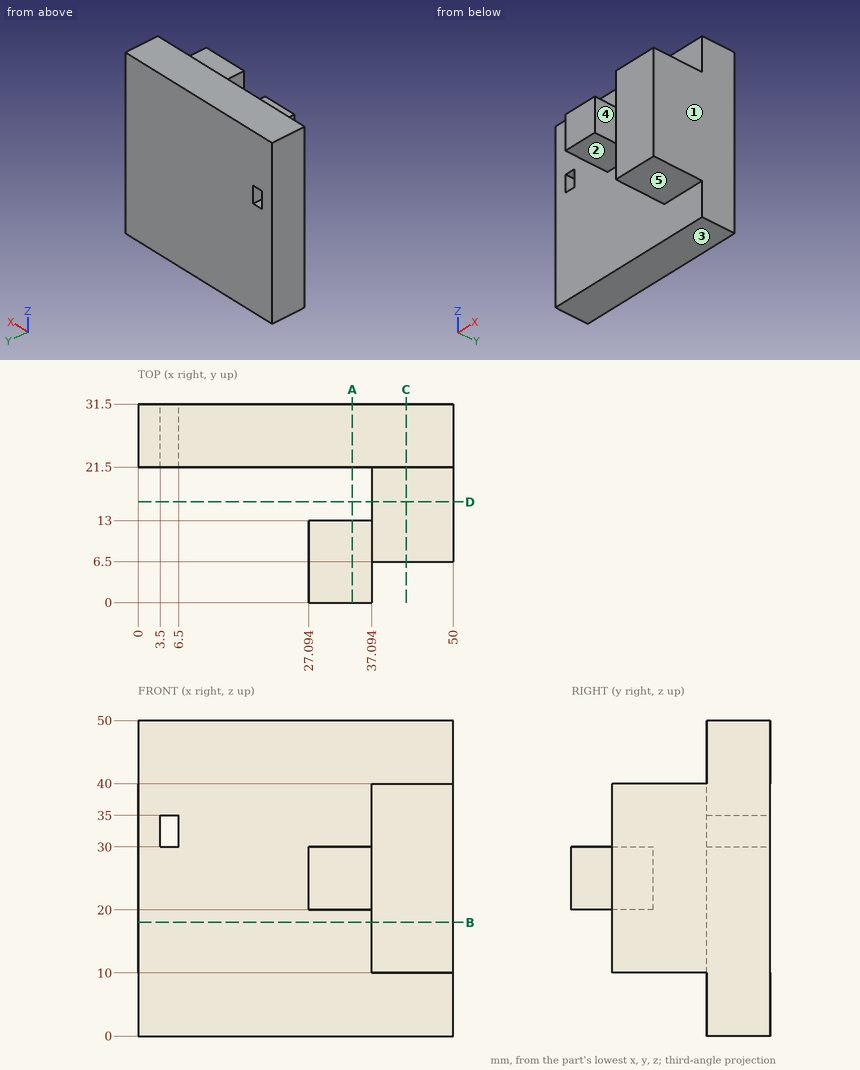
Geometry check sheet. Reference: drawing and pictorial views, mm from the part's lowest x, y, z. A direction names the side the tool comes from. Give positions to 0.01 mm unless a question says otherwise; leave off trailing zeros. Order: outer loops, then holes, each group sorted by start corner. A loop starts at its lowest first (then second) coordinate and runs counter-clockwise, first axis right, second up.
1. Access from +Z, -Z, +X, -X, +Y, -Y to the whole of each face (thin tool, end or side, straight path). Record for the marked faces 1, 2, 3, 4 and 5.
2. Section check A-A, the plane x = 34. Enter the section's corners in (y, z), and give its area (3 significant figures).
3. Gauge pin test, flat ends, axial feed: pin 1 Ø1.5 at (x, z) = (33, 19) entering from -Y; pin 2 Ø5 at (x, y) = (31, 6.5) entering from -Z; pin 3 Ø6.5 at (x, y) = (44.5, 11.5) entering from +Z; pin 4 Ø4 at (x, y) = (29.5, 28) entering from -Z. Record the tip position at first contact, or that the pin passes through.
4. Section check C-C, the plane x = 42.5. Enter the section's corners in (y, z).
5. Thickness scan on L1, parallel to X at y = 26.5, z = 34; L2, parallel to Y at x = 39, z = 9.5; L3, parallel to Z at x = 43, y = 14. Record the ranges inside material, lowest first.
6. Section check D-D, the plane y = 16. Enter the section's corners in (x, z), and give its area (3 significant figures).
7. Section check B-B, the plane z = 18. Enter the section's corners in (x, y), and give its area (3 significant figures).
Values follow:
1. face 1: +Z, -Z, +X, +Y, -Y
1. face 2: -Z, -X, -Y
1. face 3: -Z, +X, -X, +Y, -Y
1. face 4: +Z, -Z, +X, -Y
1. face 5: -Z, +X, -X, -Y
2. outline: (0, 20) - (13, 20) - (13, 30) - (0, 30) - close; (21.5, 0) - (31.5, 0) - (31.5, 50) - (21.5, 50) - close
2. area: 630 mm2
3. pin 1: stops at y = 21.5
3. pin 2: stops at z = 20
3. pin 3: stops at z = 40
3. pin 4: stops at z = 0
4. outline: (6.5, 10) - (21.5, 10) - (21.5, 0) - (31.5, 0) - (31.5, 50) - (21.5, 50) - (21.5, 40) - (6.5, 40) - close
5. L1: x = 0 to 3.5, 6.5 to 50
5. L2: y = 21.5 to 31.5
5. L3: z = 10 to 40
6. outline: (37.09, 10) - (50, 10) - (50, 40) - (37.09, 40) - close
6. area: 387 mm2
7. outline: (0, 21.5) - (37.09, 21.5) - (37.09, 6.5) - (50, 6.5) - (50, 31.5) - (0, 31.5) - close
7. area: 694 mm2
